Geometry check sheet. Reference: the model listing, model coordinates, mm. A direction names the side the tool comes from. Coordinates: 2 decimals unless noted, no trailing zeros. Order: outer loops, then holes, each group sorted by start corner. A loop starts at its lowest first (then second) coordinate and runs counter-clockwise, first axis right, second up. Notation, with made-up numbers: (-5.5, 89) - (24.5, 89) arc R12 ccw to (24.5, 106) - close; hole circle Ø3 at (51.25, 36.25). An arc over 180 degrees is marked (long way). Put each result on its own line as item: value.
Autodesk Inventor part; units mm, degrees
ref_plane "YZ Plane" through (0, 0, 0) normal (1, 0, 0) x (0, 1, 0)
ref_plane "XZ Plane" through (0, 0, 0) normal (0, 1, 0) x (-1, 0, 0)
ref_plane "XY Plane" through (0, 0, 0) normal (0, 0, 1) x (1, 0, 0)
sketch "Sketch1" plane through (0, 0, 0) normal (0, 0, 1) x (1, 0, 0)
  circle A0 centre (-1.6749, 21.9538) radius 2.1844
  circle A1 centre (-1.6749, -3.4462) radius 2.1844
  line L0 (23.7251, 85.917) -> (23.7251, -92.3462)
  line L1 (-28.6624, -92.3462) -> (-28.6624, 91.8038)
  line L2 (17.3751, 64.8163) -> (20.5501, 63.2288)
  line L3 (20.5501, 63.2288) -> (20.5501, 10.8413)
  line L4 (20.5501, 10.8413) -> (17.3751, 12.4288)
  line L5 (17.3751, 12.4288) -> (17.3751, 64.8163)
  line L6 (20.5501, 75.9288) -> (17.3751, 83.8663)
  line L7 (20.5501, 90.2163) -> (20.5501, 75.9288)
  line L8 (17.6728, 70.1741) -> (14.4978, 78.1116)
  line L9 (17.3751, 83.8663) -> (20.5501, 90.2163)
  line L10 (-18.3436, 12.4288) -> (-15.1686, 4.4913)
  line L11 (-15.9624, 17.1913) -> (-12.7874, 9.2538)
  line L12 (-15.9624, 17.1913) -> (14.4978, 78.1116)
  line L13 (-23.1061, 2.9038) -> (-19.9311, -5.0337)
  line L14 (-23.1061, 2.9038) -> (-23.1061, -11.3837)
  line L15 (-20.7249, 7.6663) -> (-18.3436, 12.4288)
  line L16 (-15.1686, 4.4913) -> (-17.5499, -0.2712)
  line L17 (-19.9311, -5.0337) -> (-23.1061, -11.3837)
  line L18 (11.8546, 90.2163) -> (11.8546, 82.3502)
  line L19 (11.8546, 90.2163) -> (-6.4374, 90.2163)
  line L20 (11.8546, 82.3502) -> (-6.4374, 45.7663)
  line L21 (0.5095, 17.1913) -> (-6.4374, 4.4913)
  line L22 (12.6126, -19.3212) -> (0.5095, 17.1913)
  line L23 (-10.761, -3.4129) -> (-19.992, -30.0754)
  line L24 (-19.992, -30.0754) -> (-17.153, -52.6587)
  line L25 (-17.153, -52.6587) -> (-9.533, -62.1837)
  line L26 (-9.533, -30.0754) -> (-1.9594, -8.2002)
  line L27 (-5.9563, -5.5321) -> (-10.761, -3.4129)
  line L28 (20.5501, -79.2004) -> (20.5501, -92.3462)
  line L29 (6.9368, -62.1837) -> (4.2652, -64.3209)
  line L30 (-1.5433, -71.7065) -> (14.9685, -92.3462)
  arc A2 (-1.5433, -71.7065) -> (3.0742, -66.8586) centre (-1.6875, -66.9462) ccw
  circle A3 centre (-1.6875, -66.9462) radius 2.1844
  arc A4 (4.2652, -64.3209) -> (3.0742, -66.8586) centre (6.2486, -66.8002) ccw
  line L31 (20.5501, -79.2004) -> (6.9368, -62.1837)
  line L32 (23.7251, -92.3462) -> (20.5501, -92.3462)
  circle A5 centre (-1.6749, -54.2462) radius 2.1844
  arc A6 (-4.5442, -50.4451) -> (-5.5294, -57.0433) centre (-1.6749, -54.2462) ccw
  line L33 (-9.533, -62.1837) -> (-5.8225, -59.2153)
  line L34 (0.5075, -54.1513) -> (0.5095, -54.1497)
  line L35 (0.5095, -54.1497) -> (0.5073, -54.1469)
  line L36 (-4.2611, -48.1864) -> (-7.1105, -44.6247)
  arc A7 (-4.5442, -50.4451) -> (-4.2611, -48.1864) centre (-5.5007, -49.1781) ccw
  arc A8 (-5.8225, -59.2153) -> (-5.5294, -57.0433) centre (-6.8142, -57.9757) ccw
  arc A9 (-4.5324, 25.7638) -> (-6.4374, 21.9538) centre (-1.6749, 21.9538) ccw
  line L37 (17.6728, 70.1741) -> (-4.5324, 25.7638)
  line L38 (-6.4374, 21.9538) -> (-12.7874, 9.2538)
  line L39 (-6.4374, 4.4913) -> (-3.5794, 0.9189)
  line L40 (2.1657, -6.2625) -> (12.6126, -19.3212)
  arc A10 (2.1657, -6.2625) -> (-3.5794, 0.9189) centre (-1.6749, -3.4462) ccw
  arc A11 (-5.9563, -5.5321) -> (-1.9594, -8.2002) centre (-1.6749, -3.4462) ccw
  line L41 (14.9685, -92.3462) -> (44.3118, -92.3462) construction
  line L42 (-2.7748, -92.3462) -> (14.9685, -92.3462)
  line L43 (-28.6624, -92.3462) -> (-23.2121, -92.3462)
  line L44 (-18.5725, -92.3462) -> (-28.6624, -92.3462)
  line L45 (-20.7249, 7.6663) -> (-17.5499, -0.2712)
  line L46 (-28.6624, 98.1538) -> (-28.6624, 101.3288)
  line L47 (-19.1374, 101.3288) -> (11.0251, 101.3288)
  line L48 (23.7251, 90.2163) -> (23.7251, 85.917)
  line L49 (11.0251, 101.3288) -> (23.7251, 90.2163)
  arc A12 (-19.1374, 101.3288) -> (-28.6624, 91.8038) centre (-19.1374, 91.8038) ccw
  arc A13 (-6.4374, 74.6137) -> (-6.4374, 83.5939) centre (-8.0249, 79.1038) ccw
  circle A14 centre (-8.0249, 79.1038) radius 2.1844
  line L50 (-6.4374, 90.2163) -> (-6.4374, 83.5939)
  line L51 (-18.5725, -92.3462) -> (-15.3911, -92.3462)
  line L52 (-15.3911, -92.3462) -> (-15.3911, -76.5759)
  line L53 (-15.3911, -76.5759) -> (-2.7748, -92.3462)
  arc A15 (-6.4374, 49.4405) -> (-6.4374, 58.4207) centre (-8.0249, 53.9306) ccw
  circle A16 centre (-8.0249, 53.9306) radius 2.1844
  line L54 (-6.4374, 74.6137) -> (-6.4374, 58.4207)
  line L55 (-6.4374, 49.4405) -> (-6.4374, 45.7663)
  line L56 (-1.6749, -54.2462) -> (17.3751, -54.2462) construction
  circle A17 centre (-8.0249, -35.1962) radius 2.0955
  arc A18 (-9.4376, -30.6481) -> (-7.8877, -39.9567) centre (-8.0249, -35.1962) ccw
  line L57 (-9.4376, -30.6481) -> (-9.533, -30.0754)
  line L58 (-7.1105, -44.6247) -> (-7.8877, -39.9567)
  point P0 (0, 0)
  point P1 (2.838, -65.4627)
  point P2 (-4.4495, -58.1169)
  point P3 (-3.0588, -49.6892)
  dimension "d0" = 4.3688
  dimension "d1" = 4.3688
  dimension "d3" = 9.525
  dimension "d4" = 4.3688
  dimension "d5" = 3.175
  dimension "d6" = 9.525
  dimension "d7" = 1.5875
  dimension "d8" = 9.525
  dimension "d14" = 3.175
  dimension "d15" = 9.525
  dimension "d18" = 9.525
  dimension "d19" = 4.3688
  dimension "d20" = 3.1814
  dimension "d22" = 9.525
  dimension "d23" = 4.3688
  dimension "d27" = 4.191
  dimension "d28" = 9.525
extrude "Extrusion1" add sketch "Sketch1" along normal blind 1.5875
equation "\"BendRadius\" = Thickness"
equation "\"BendReliefWidth\" = Thickness"
equation "\"BendReliefDepth\" = 0.5 * Thickness"
equation "\"CornerReliefSize\" = 4 * Thickness"
equation "\"MinimumRemnant\" = 2 * Thickness"
equation "\"TransitionRadius\" = BendRadius"
equation "\"JacobiRadiusSize\" = BendRadius"
equation "\"GapSize\" = Thickness"
properties part number "sideplate" material "Acetal Resin, White"
Q1. Access from +Z, -Z, +X, -X, +Y, -Y to the whole of each face (thin tool, end or side, straight path). Record for faces 5 (the flat face through (13.84, -70.81, 0.78)), 6 (the flat face through (17.286, 95.85, 0.783)).
Answer block:
face 5: +Z, -Z
face 6: +Z, -Z, +X, +Y
Q2. Depth check by flat-ended pin: pin 1 Ø2.5 at (x, y) = (-8.02, 79.1) entering from -Z. Enter the tip coordinate at first touch or a pass-through.
Answer block:
pin 1: passes through
Q3. Section check C-C on z = 1. State how many separate pieces and enclosed holes the cut face has, then the cut area to 3 significant figures.
Answer block:
separate pieces: 1
enclosed holes: 15
area: 7,680 mm^2
Q4. Thickness scan on L1, parallel to X at y = 20.5, z = 0.55; L2, parallel to X at y = -11, z = 0.45; L3, parallel to X at y = 7.5, z = 0.2. Record the ranges inside material, lowest first. Write a range as [from, to].
Answer block:
L1: x = [-28.66, -14.31], [-7.16, -3.31], [-0.04, 17.38], [20.55, 23.73]
L2: x = [-28.66, -23.11], [-22.91, -13.39], [-2.93, 5.96], [9.85, 23.73]
L3: x = [-28.66, -20.66], [-16.37, -4.79], [3.72, 23.73]
Q5. Draft check along Y on faces 1 (the flat face through (6.597, -81.882, 0.783)), 2 (the cylindrical face through (-8.31, 76.94, 0.78)), 3 (the flat face through (-9, 6, 1.588)), 4 (the cylindrical face through (-25.95, 98.46, 0.78)). Enter one of: pulls with the +Y half, pulls with the -Y half, needs draft (parallel to the pull), parting line crosses it, or undercut.
Answer block:
face 1: undercut
face 2: undercut
face 3: needs draft
face 4: pulls with the +Y half
Q6. Section check B-B on y = -24. Record the boundary of the cut face in (x, z), then the cut area to 3 significant figures.
Answer block:
outline: (-28.66, 0) - (-17.89, 0) - (-17.89, 1.59) - (-28.66, 1.59) - close; (-7.43, 0) - (23.73, 0) - (23.73, 1.59) - (-7.43, 1.59) - close
area: 66.6 mm^2
Q7. Section check A-A on x = 9. Record the boundary of the cut face in (y, z).
Answer block:
outline: (-92.35, 0) - (-84.89, 0) - (-84.89, 1.59) - (-92.35, 1.59) - close; (-64.76, 0) - (-14.81, 0) - (-14.81, 1.59) - (-64.76, 1.59) - close; (-8.42, 0) - (52.83, 0) - (52.83, 1.59) - (-8.42, 1.59) - close; (67.12, 0) - (76.64, 0) - (76.64, 1.59) - (67.12, 1.59) - close; (90.22, 0) - (101.33, 0) - (101.33, 1.59) - (90.22, 1.59) - close
